Work out the finished part from the listing and answer in its coordinate system (mm). A direction names the side the tool comes from. Coordinates: 2 decimals unless noted, no trailing zeros. Loops run counter-clockwise (first coordinate to the right, second up) from the corner with the lowest first, then second, coordinate; pieces in that order, holes last. Notation, with made-up numbers: (23, -17) -> (63, -17) arc R27 ccw to (63, 20) -> close; hole circle Ø7 at (-24, 37). An arc over 180 degrees is marked (long way). Use a Markdown table: item, result. Add a question column.
```python
from build123d import *

# Parameters (mm, degrees)
F0_R     = 4.5
F1_DEPTH = 1.5
F2_R     = 3.5
F3_DEPTH = 5
F4_R     = 1.9
F5_DEPTH = 25


with BuildPart() as f1:
    # F0 (on Top) → F1 (new body)
    with BuildSketch(Plane.XY):
        Circle(F0_R)
    extrude(amount=F1_DEPTH)

    # F2 (on face) → F3 (join)
    with BuildSketch(Plane.XY.offset(1.5)):
        Circle(F2_R)
    extrude(amount=F3_DEPTH)

    # F4 (on Top) → F5 (cut)
    with BuildSketch(Plane.XY):
        Circle(F4_R)
    extrude(amount=F5_DEPTH, mode=Mode.SUBTRACT)


solid = f1.part
```
Item 1: For a pull along X with two mould halves and no side action, classify faces 3 (the face through (2, -1, 0)), 4 (the face through (3.233, -1.341, 3.965)), 5 (the face through (-1.9, 0.08, 3.2)) as +X half, -X half, draft (parallel to the pull), parting line (faces both ways), or undercut.
Item 2: Section A-A (x = 0) is taken. Determine the outline of the cut face in (y, z), then the cut area to 3 significant figures.
Item 3: Section D-D (y = -2.5) is taken. Determine the outline of the cut face in (x, z), then the cut area to 3 significant figures.
Item 4: Section C-C (z = 1.75) is taken. Determine the outline of the cut face in (x, y), then the cut area to 3 significant figures.
Item 5: For faces 1 (the face through (2, -2, 6.5)), 2 (the face through (0, -4, 1.5)), determine the directions among +Z, -Z, +X, -X, +Y, -Y from which every point of the face is accessible in a straight line to the end or side of a thin tool.
Item 6: Given pin 1 (2 mm diameter, centred on x = -2.5, z = 5.5, fed in from -Y); pin 2 (2 mm diameter, centred on y = -0.5, z = 3.5, fed in from +X); pin 3 (2 mm diameter, centred on x = 0, z = 5.5, fed in from +Y), each flat-ended and moving along its own axis, determine where each tip first touches the part or whether it passes through.
Item 7: Find the intervals of material crossed by probe 1 along Y at (x, z) = (0, 5.25); probe 2 along Z at (x, y) = (3.5, -1.5); probe 3 along X at (y, z) = (1.5, 2.75), in increasing order.
Output:
| question | item | result |
|---|---|---|
| 1 | face 3 | draft |
| 1 | face 4 | parting line |
| 1 | face 5 | undercut |
| 2 | outline | (-4.5, 0) -> (-1.9, 0) -> (-1.9, 6.5) -> (-3.5, 6.5) -> (-3.5, 1.5) -> (-4.5, 1.5) -> close; (1.9, 0) -> (4.5, 0) -> (4.5, 1.5) -> (3.5, 1.5) -> (3.5, 6.5) -> (1.9, 6.5) -> close |
| 2 | area | 23.8 mm2 |
| 3 | outline | (-3.74, 0) -> (3.74, 0) -> (3.74, 1.5) -> (2.45, 1.5) -> (2.45, 6.5) -> (-2.45, 6.5) -> (-2.45, 1.5) -> (-3.74, 1.5) -> close |
| 3 | area | 35.7 mm2 |
| 4 | outline | circle Ø7 at (0, 0); hole circle Ø3.8 at (0, 0) |
| 4 | area | 27.1 mm2 |
| 5 | face 1 | +Z, +X, -X, +Y, -Y |
| 5 | face 2 | +Z |
| 6 | pin 1 | stops at y = -3.16 |
| 6 | pin 2 | stops at x = 3.5 |
| 6 | pin 3 | stops at y = 3.5 |
| 7 | probe 1 | y = -3.5 to -1.9, 1.9 to 3.5 |
| 7 | probe 2 | z = 0 to 1.5 |
| 7 | probe 3 | x = -3.16 to -1.17, 1.17 to 3.16 |
